Geometry check sheet. Reference: the model listing, model coordinates, mm. Coordinates: 2 decimals unless noted, no trailing zeros. Write each loop counter-clockwise with the first axis right and the second up, starting at its lowest first coordinate (ties: lowest second). Pieces come first, ordered by that corner, then holes. Notation, with made-up numbers: (-33, -3.5) -> (2, -3.5) arc R20 ccw to (2, 9.5) -> close; hole circle Ø7 at (-19.5, -33.75). An arc over 180 degrees is marked (long way). One line per question, with ' | ' between items.
from build123d import *

# Parameters (mm, degrees)
F0_W     = 25.7850475609
F0_H     = 69.0255090594
F1_DEPTH = 97.1566960216
F2_W     = 29.3421596289
F2_H     = 68.0039366707
F3_DEPTH = 74.8365670443
F5_W     = 27.3843407631
F5_H     = 64.3117055297


with BuildPart() as f1:
    # F0 (on Top) → F1 (new body)
    with BuildSketch(Plane.XY):
        with Locations((44.0845470876, 10.3604607284)):
            Rectangle(F0_W, F0_H)
    extrude(amount=F1_DEPTH)

    # F2 (on face) → F3 (join)
    with BuildSketch(Plane.YZ.offset(56.977070868)):
        with Locations((14.6710798144, 47.3301787861)):
            Rectangle(F2_W, F2_H)
    extrude(amount=-F3_DEPTH)


with BuildPart() as f6:
    # F5 (on Top) → F6 (revolve)
    with BuildSketch(Plane.XY):
        with Locations((-27.3843705654, 0.8298419416)):
            Rectangle(F5_W, F5_H)
    revolve(axis=Axis((-13.6922001839, 0.8298419416, 0), (0, -1, 0)))


solid = f6.part
1. Go/stop test with flat-tipped pins: P1, Ø4, axis at y = -23, z = -3, coming from the -X side; P2, Ø4, axis at x = -9, y = 17.5, coming from the -Z side; P3, Ø5, axis at x = -17.5, y = 21, coming from the -Z side. Record where each tip stops, or that it passes through.
Worked answers:
P1: x = -41.06 | P2: z = -27.25 | P3: z = -27.35
2. Cross-section at C-C on z = 16.5. Record the boundary of the cut face in (x, y), and give its area (3 significant figures).
Worked answers:
outline: (-35.55, -31.33) -> (8.16, -31.33) -> (8.16, 32.99) -> (-35.55, 32.99) -> close | area: 2,810 mm²
3. Cross-section at A-A on y = 23. Record the boundary of the cut face in (x, z), and give its area (3 significant figures).
Worked answers:
outline: circle Ø54.77 at (-13.69, 0) | area: 2,360 mm²
4. Cross-section at B-B on x = -34.5. Record the boundary of the cut face in (y, z), and give its area (3 significant figures).
Worked answers:
outline: (-31.33, -17.8) -> (32.99, -17.8) -> (32.99, 17.8) -> (-31.33, 17.8) -> close | area: 2,290 mm²
5. Material ranges on line 1 (Z direction, x = -14, y = -17); line 2 (X direction, y = 2, z = -11); line 3 (Z direction, x = -37.5, y = -16.5), recorded low to high. Write a range as from..to.
Worked answers:
line 1: -27.38..27.38 | line 2: -38.77..11.39 | line 3: -13.53..13.53
6. Mould release check, pull along X, two halves, no side actions. Record for faces 1 (the face through (6.5, 1.3, -18.5)), 2 (the face through (-13, 32.986, 0)): released by +X, released by -X, zero draft, split by the parting line, or undercut.
Worked answers:
face 1: split by the parting line | face 2: zero draft
